from build123d import *

# Parameters (mm, degrees)
F0_W      = 38.1
F0_H      = 25.4
F3_DEPTH  = 73.8923922181
F5_DEPTH  = 25.4
F7_DEPTH  = 25.4
F9_DEPTH  = 25.4
F11_DEPTH = 25.4
F13_DEPTH = 25.4


# Not quite as in the source:
# - ends of sketch curves that miss each other by under 0.0002 mm in the source are joined


with BuildPart() as f1:
    # F0 (on Front) → F1 (revolve)
    with BuildSketch(Plane.XZ):
        with Locations((19.05, 12.7)):
            Rectangle(F0_W, F0_H)
    revolve(axis=Axis((0, 0, 12.7), (0, 0, -1)))

    # F2 (on Top) → F3 (cut)
    with BuildSketch(Plane.XY):
        Polygon((-19.3802006543, 13.6906001717), (0, -21.8694005162), (17.7799984813, 13.6905994838), align=None)
    extrude(amount=F3_DEPTH, mode=Mode.SUBTRACT)

    # F4 (on face) → F5 (cut)
    with BuildSketch(Plane(origin=(0, 0, 0), x_dir=(1, 0, 0), z_dir=(0, 0, -1))):
        Polygon((-9.8248589784, 21.8694005162), (-23.8991640508, 21.8694005162), (-23.8595362753, 20.1035637146), (-15.7059820649, 20.1035637146), (-23.725675419, 14.439499937), (-23.725675419, 11.4520248026), (-10.8296805993, 11.4520248026), (-10.8296805993, 13.090708293), (-22.2545247525, 13.090708293), align=None)
    extrude(amount=-F5_DEPTH, mode=Mode.SUBTRACT)

    # F6 (on face) → F7 (cut)
    with BuildSketch(Plane(origin=(0, 0, 0), x_dir=(1, 0, 0), z_dir=(0, 0, -1))):
        Polygon((15.7712604851, 27.6608336717), (10.5691235512, 18.2647015899), (13.062780723, 18.0983748287), (15.1800094172, 21.327663213), (16.9541146606, 18.1070137769), (19.2498695105, 18.1070137769), align=None)
    extrude(amount=-F7_DEPTH, mode=Mode.SUBTRACT)

    # F8 (on face) → F9 (cut)
    with BuildSketch(Plane(origin=(0, 0, 0), x_dir=(1, 0, 0), z_dir=(0, 0, -1))):
        Polygon((2.8216354549, -20.8048354834), (2.9142363928, -19.2329455167), (-3.8865676615, -19.2329455167), (-3.8865676615, -25.3260713071), (2.5894464925, -25.3260713071), (2.5894464925, -23.6380007118), (-2.1816743538, -23.6380007118), (-2.1816743538, -20.8048354834), align=None)
    extrude(amount=-F9_DEPTH, mode=Mode.SUBTRACT)

    # F10 (on face) → F11 (cut)
    with BuildSketch(Plane(origin=(0, 0, 0), x_dir=(1, 0, 0), z_dir=(0, 0, -1))):
        with BuildLine():
            ThreePointArc((5.8152880434, 37.6535844904), (0, 38.1), (-5.8152880434, 37.6535844904))
            ThreePointArc((-5.8152880434, 37.6535844904), (0, 32.267602394), (5.8152880434, 37.6535844904))
        make_face()
        with BuildLine():
            ThreePointArc((5.8152880434, 37.6535844904), (5.8281186457, 37.8766283677), (5.832397606, 38.1))
            ThreePointArc((5.832397606, 38.1), (-0.2233716323, 43.9281186457), (-5.8152880434, 37.6535844904))
            ThreePointArc((-5.8152880434, 37.6535844904), (0, 38.1), (5.8152880434, 37.6535844904))
        make_face()
    extrude(amount=-F11_DEPTH, mode=Mode.SUBTRACT)

    # F12 (on face) → F13 (join)
    with BuildSketch(Plane(origin=(0, 0, 0), x_dir=(1, 0, 0), z_dir=(0, 0, -1))):
        with BuildLine():
            ThreePointArc((-3.9919458032, -37.8902938588), (0, -38.1), (3.9919458032, -37.8902938588))
            ThreePointArc((3.9919458032, -37.8902938588), (0, -34.1025498176), (-3.9919458032, -37.8902938588))
        make_face()
        with BuildLine():
            ThreePointArc((-3.9919458032, -37.8902938588), (-0.1048891842, -42.0960738507), (3.9974501824, -38.1))
            ThreePointArc((3.9974501824, -38.1), (3.9960738507, -37.9951108158), (3.9919458032, -37.8902938588))
            ThreePointArc((3.9919458032, -37.8902938588), (0, -38.1), (-3.9919458032, -37.8902938588))
        make_face()
    extrude(amount=-F13_DEPTH)


solid = f1.part
Geometry check sheet. Reference: the model listing, model coordinates, mm. Give positions to 0.01 mm unless a question says otherwise; leave off trailing zeros. Write each loop counter-clockwise with the first axis right and the second up, starting at its lowest first coordinate (ties: lowest second). Pieces come first, ordered by that corner, then holes. Notation, with made-up numbers: (19, -5) - (60, -5) arc R28 cw to (60, 34) - close; hole circle Ø6 at (-29.5, 82). An arc over 180 degrees is marked (long way). Put each result on its own line as item: value.
1. Thickness scan on line 1 (Y direction, x = -16, z = 2.5); line 2 (Y direction, x = 15, z = 20.5); line 3 (X direction, y = 0.5, z = 14.25). Record the ranges inside material, lowest first.
Ans:
line 1: y = -34.58 to -21.87, -20.1 to -19.9, -17.51 to -13.09, -11.45 to 7.49, 13.69 to 34.58
line 2: y = -35.02 to -26.27, -21.05 to 8.13, 13.69 to 35.02
line 3: x = -38.1 to -12.19, 11.18 to 38.1
2. Sectioned sample at D-D, the plane x = 9. Enter the section's corners in (y, z), plus the area to 3 significant figures.
Ans:
outline: (-37.02, 0) - (-3.87, 0) - (-3.87, 25.4) - (-37.02, 25.4) - close; (13.69, 0) - (37.02, 0) - (37.02, 25.4) - (13.69, 25.4) - close
area: 1,430 mm²
3. Sectioned sample at C-C, the plane z = 9.75. Give the number of separate pieces and of enclosed holes in the cut face, plus the area to 3 significant figures.
Ans:
separate pieces: 1
enclosed holes: 4
area: 3,750 mm²
4. Draft check along Y on faces 1 (the flat face through (9, -7, 0)), 2 (the cylindrical face through (-0.12, -32.27, 12.52)), 3 (the flat face through (-1, 13.691, 13)). Enter one of: +Y half, -Y half, draft (parallel to the pull), parting line (faces both ways), or undercut.
Ans:
face 1: draft
face 2: -Y half
face 3: undercut
5. Go/stop test with flat-tipped pins: pin 1 (2.5 mm diameter, centred on x = 1.5, z = 10, fed in from +Y); pin 2 (0.8 mm diameter, centred on y = -12.5, z = 8.5, fed in from -X); pin 3 (2 mm diameter, centred on y = 3, z = 20, fed in from -X). Record where each tip stops, or that it passes through.
Ans:
pin 1: stops at y = 42.09
pin 2: stops at x = -36.13
pin 3: stops at x = -38.05
6. Sectioned sample at B-B, the plane y = 8.5. Enter the section's corners in (x, z).
Ans:
outline: (-37.14, 0) - (-16.55, 0) - (-16.55, 25.4) - (-37.14, 25.4) - close; (15.18, 0) - (37.14, 0) - (37.14, 25.4) - (15.18, 25.4) - close
7. Sectioned sample at A-A, the plane x = -17. Enter the section's corners in (y, z).
Ans:
outline: (-34.1, 0) - (-21.87, 0) - (-21.87, 25.4) - (-34.1, 25.4) - close; (-20.1, 0) - (-19.19, 0) - (-19.19, 25.4) - (-20.1, 25.4) - close; (-16.8, 0) - (-13.09, 0) - (-13.09, 25.4) - (-16.8, 25.4) - close; (-11.45, 0) - (9.32, 0) - (9.32, 25.4) - (-11.45, 25.4) - close; (13.69, 0) - (34.1, 0) - (34.1, 25.4) - (13.69, 25.4) - close
